Autodesk Fusion 360 part; units mm, degrees
sketch "Sketch3" plane through (0, 0, 0) normal (0, 0, 1) x (1, 0, 0)
  arc A0 (12.1503, 52.1262) -> (-13.4843, 51.7971) centre (-0.5229, 40.7362) ccw
  arc A1 (42.8137, 32.1209) -> (22.965, 48.3464) centre (25.7842, 31.5419) ccw
  arc A2 (53.4441, -2.9141) -> (48.6687, 22.2739) centre (40.0266, 7.5887) ccw
  arc A3 (39.0674, -36.5855) -> (51.5997, -14.2208) centre (35.5401, -19.9153) ccw
  arc A4 (6.4107, -53.1382) -> (30.3867, -44.0615) centre (14.424, -38.1007) ccw
  arc A5 (-29.2457, -44.8269) -> (-5.0446, -53.2853) centre (-13.4412, -38.4584) ccw
  arc A6 (-51.2177, -15.5406) -> (-38.1155, -37.5763) centre (-35.0172, -20.821) ccw
  arc A7 (-24.1984, 47.741) -> (-43.6241, 31.0114) centre (-26.5853, 30.8696) ccw
  arc A8 (-49.2244, 21.0173) -> (-53.3517, -4.2849) centre (-40.2082, 6.5588) ccw
  arc A9 (-49.2244, 21.0173) -> (-43.6241, 31.0114) centre (-55.5183, 31.1103) ccw
  arc A10 (-24.1984, 47.741) -> (-13.4843, 51.7971) centre (-22.5322, 59.5183) ccw
  arc A11 (12.1503, 52.1262) -> (22.965, 48.3464) centre (20.997, 60.0771) ccw
  arc A12 (42.8137, 32.1209) -> (48.6687, 22.2739) centre (54.7014, 32.5251) ccw
  arc A13 (53.4441, -2.9141) -> (51.5997, -14.2208) centre (62.8105, -10.2457) ccw
  arc A14 (39.0674, -36.5855) -> (30.3867, -44.0615) centre (41.5298, -48.2225) ccw
  arc A15 (6.4107, -53.1382) -> (-5.0446, -53.2853) centre (0.8168, -63.6354) ccw
  arc A16 (-29.2457, -44.8269) -> (-38.1155, -37.5763) centre (-40.2783, -49.2726) ccw
  arc A17 (-51.2177, -15.5406) -> (-53.3517, -4.2849) centre (-62.5268, -11.8546) ccw
  dimension "d14" = 11.8946
extrude "Extrude1" add sketch "Sketch3" along normal blind 10
Part model, mm, in its own coordinate system. Round coordinates to 2 decimals unless told otherwise and drop trailing zeros. Loops run counter-clockwise (first coordinate to the right, second up) from the corner with the lowest first, then second, coordinate; pieces in that order, holes last.
Item 1: Drop flat-ended pins along their axis: P1, Ø4, axis at x = -0.5, z = 3.5, coming from the -Y side; P2, Ø3, axis at y = 33, z = 8.5, coming from the -X side; P3, Ø6, axis at x = -29, z = 7, coming from the -Y side. Give the stop position or say it passes through.
Item 2: Cut at B-B, the plane x = 10.5. Give the cut face in (y, z), then the cut area to 3 significant figures.
Item 3: Cut at A-A, the plane z = 7. Give the cut face in (x, y) (1 decimal), then the cut area to 3 significant figures.
Item 4: Drill centre lines: line 1 (Y direction, x = 17.5, z = 8.75); line 2 (X direction, y = -23, z = 8.5); line 3 (X direction, y = -39, z = 3). Where is each one in solid material? Low to high.
Item 5: Mould opens along Y. For faces 1 (the face through (44.521, 26.374, 4.93)), 2 (the face through (-1, 2, 10)), 3 (the face through (51.06, -8.41, 4.93)), 4 (the face through (-49.56, -29.7, 4.93)) say: +Y half, -Y half, draft (parallel to the pull), parting line (faces both ways), or undercut.
Item 6: Cut at C-C, the plane y = 25. Give the cut face in (x, z).
A:
1. P1: stops at y = -52.21
1. P2: stops at x = -43.61
1. P3: stops at y = -49.97
2. outline: (-54.68, 0) - (53.73, 0) - (53.73, 10) - (-54.68, 10) - close
2. area: 1,080 mm2
3. outline: (-53.4, -4.3) arc R11.9 cw to (-51.2, -15.5) arc R17 ccw to (-38.1, -37.6) arc R11.9 cw to (-29.2, -44.8) arc R17 ccw to (-5, -53.3) arc R11.9 cw to (6.4, -53.1) arc R17 ccw to (30.4, -44.1) arc R11.9 cw to (39.1, -36.6) arc R17 ccw to (51.6, -14.2) arc R11.9 cw to (53.4, -2.9) arc R17 ccw to (48.7, 22.3) arc R11.9 cw to (42.8, 32.1) arc R17 ccw to (23, 48.3) arc R11.9 cw to (12.2, 52.1) arc R17 ccw to (-13.5, 51.8) arc R11.9 cw to (-24.2, 47.7) arc R17 ccw to (-43.6, 31) arc R11.9 cw to (-49.2, 21) arc R17 ccw to start
3. area: 9,570 mm2
4. line 1: y = -54.86 to 48.71
4. line 2: x = -51.92 to 52.3
4. line 3: x = -34.28 to 34.02
5. face 1: +Y half
5. face 2: draft
5. face 3: undercut
5. face 4: undercut
6. outline: (-45.31, 0) - (45.49, 0) - (45.49, 10) - (-45.31, 10) - close
